Drawing for the job (mm, zero at the part's lowest x, y, z). Round coordinates to 2 decimals unless told otherwise and drop trailing zeros. Write each loop counter-clockwise with the first axis right and the second up, starting at its lowest first coordinate (ties: lowest second). Pieces come first, ordered by that corner, then holes.
Item 1: Drop flat-ended pins along their axis: pin 1 Ø6 at (x, y) = (26.5, 25.5) entering from +Z; pin 2 Ø2 at (x, y) = (25.5, 9) entering from -Z. Give the stop position or say it passes through.
Item 2: Wall check: probe 1 along Y at (x, z) = (30, 42); probe 2 along Z at (x, y) = (38.5, 27); probe 3 along X at (y, z) = (26, 36). Give the ranges that are in metal, low to high.
Item 3: Band-saw the part on B-B, the plane x = 30. Write the cut outline in (y, z), then the cut area to 3 significant figures.
Item 4: Band-saw the part on A-A, the plane z = 36.5. Write the cut outline in (x, y), then the cut area to 3 significant figures.
Item 5: Mould opens along Y. For the marked faces 1, 2 and 3 say: +Y half, -Y half, draft (parallel to the pull), parting line (faces both ways), or undercut.
Item 6: Band-saw the part on C-C, the plane y = 25. Write the cut outline in (x, z).
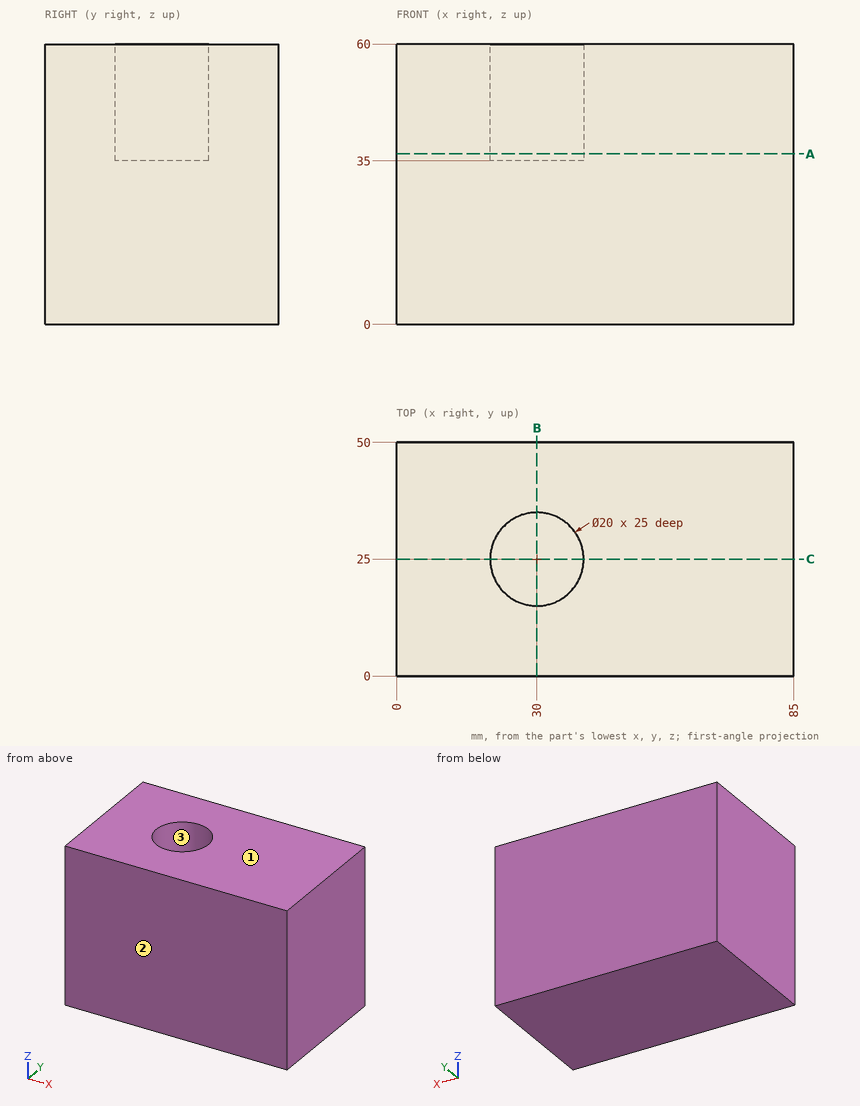
Results:
1. pin 1: stops at z = 35
1. pin 2: stops at z = 0
2. probe 1: y = 0 to 15, 35 to 50
2. probe 2: z = 0 to 35
2. probe 3: x = 0 to 20.05, 39.95 to 85
3. outline: (0, 0) - (50, 0) - (50, 60) - (35, 60) - (35, 35) - (15, 35) - (15, 60) - (0, 60) - close
3. area: 2,500 mm2
4. outline: (0, 0) - (85, 0) - (85, 50) - (0, 50) - close; hole circle Ø20 at (30, 25)
4. area: 3,940 mm2
5. face 1: draft
5. face 2: -Y half
5. face 3: undercut
6. outline: (0, 0) - (85, 0) - (85, 60) - (40, 60) - (40, 35) - (20, 35) - (20, 60) - (0, 60) - close
